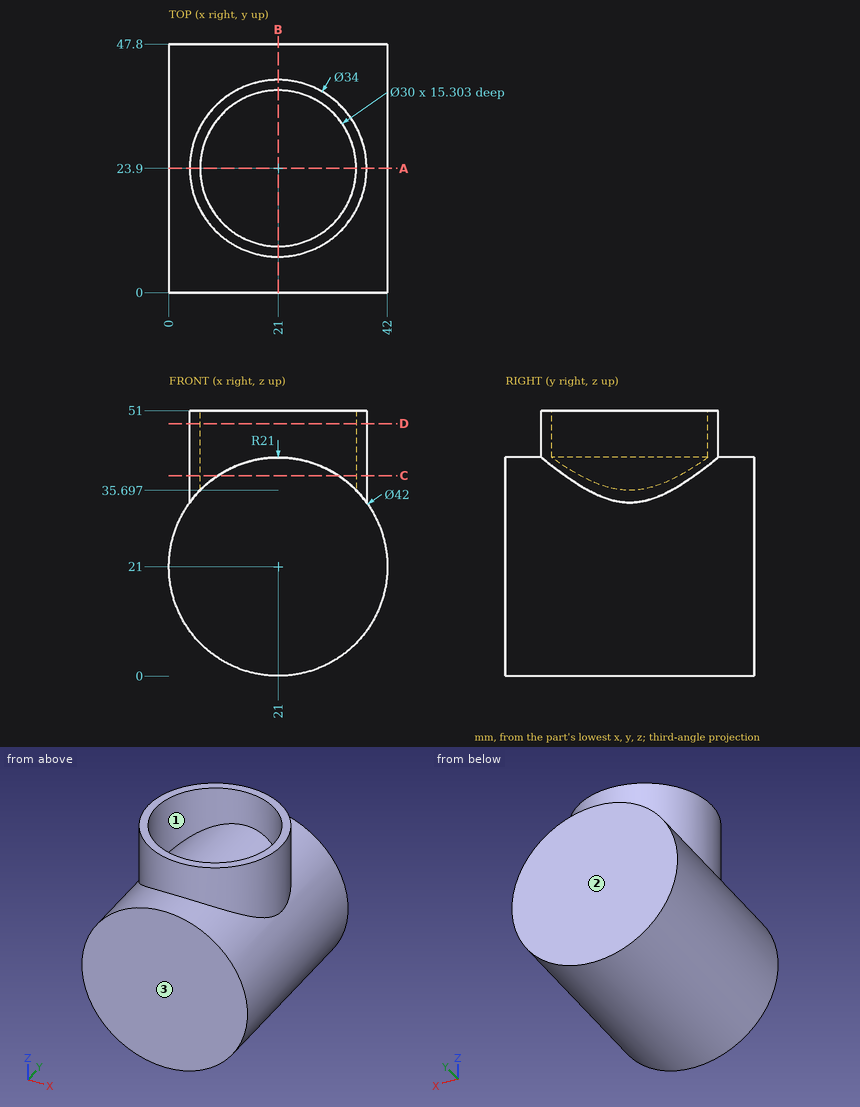
Design review of the part shown in the three views and the two pictorial views. Dimensions are in mm from the part's minimum x, y and z. Round coordinates to 2 decimals unless told otherwise and drop trailing zeros. Loops run counter-clockwise (first coordinate to the right, second up) from the corner with the lowest first, then second, coordinate; pieces in that order, holes last. Notation, with made-up numbers: (41.25, -19) -> (79.25, -19) arc R31 ccw to (79.25, 15) -> close; hole circle Ø8 at (-9, -14). An arc over 180 degrees is marked (long way). Use one line per item in the form item = value. Start each with the question number.
Q1. Wall thickness on line 1 along Y through (x, z) = (21, 43); line 2 along X through (y, z) = (18, 39); line 3 along Y through (x, z) = (32, 41): over which ranges is each line inside the solid? List them lowest first. Write a range as [from, to].
Q2. For pin 1 Ø2 at (x, y) = (6, 41.5) entering from +Z; pin 2 Ø1.5 at (y, z) = (35, 14.5) entering from +X; pin 3 Ø2 at (y, z) = (16, 34.5) entering from +X, all flat-tipped, find the tip position at first contact; note any pin that passes through.
Q3. We need section C-C on z = 38.5. Give the boundary of the cut face in (x, y), then the cut area to 3 significant figures.
Q4. We need section D-D on z = 48.5. Give the boundary of the cut face in (x, y), then the cut area to 3 significant figures.
Q5. Draft analysis for pull direction Y (two halves, no side actions). For the marked faces 1, 2 and 3, state which applies: +Y half, -Y half, draft (parallel to the pull), parting line (faces both ways), or undercut.
Q6. We need section A-A on y = 23.9. Give the boundary of the cut face in (x, z), then the cut area to 3 significant figures.
Q7. We need section B-B on x = 21. Give the boundary of the cut face in (y, z).
Calculated:
q1.line_1 = [6.9, 8.9], [38.9, 40.9]
q1.line_2 = [5.06, 7.21], [10.18, 31.82], [34.79, 36.94]
q1.line_3 = [10.94, 13.7], [34.1, 36.86]
q2.pin_1 = 36.65
q2.pin_2 = 41.2
q2.pin_3 = 37.87
q3.outline = (9.39, 0) -> (32.61, 0) -> (32.61, 11.48) arc R17 ccw to (32.61, 36.32) -> (32.61, 47.8) -> (9.39, 47.8) -> (9.39, 36.32) arc R17 ccw to (9.39, 11.48) -> close; hole (9.39, 14.4) -> (9.39, 33.4) arc R15 ccw to start; hole (32.61, 14.4) arc R15 ccw to (32.61, 33.4) -> close
q3.area = 1,210 mm²
q4.outline = circle Ø34 at (21, 23.9); hole circle Ø30 at (21, 23.9)
q4.area = 201 mm²
q5.face_1 = undercut
q5.face_2 = +Y half
q5.face_3 = -Y half
q6.outline = (4, 33.33) arc R21 ccw (long way) to (38, 33.33) -> (38, 51) -> (36, 51) -> (36, 35.7) arc R21 ccw to (6, 35.7) -> (6, 51) -> (4, 51) -> close
q6.area = 1,450 mm²
q7.outline = (0, 0) -> (47.8, 0) -> (47.8, 42) -> (40.9, 42) -> (40.9, 51) -> (38.9, 51) -> (38.9, 42) -> (8.9, 42) -> (8.9, 51) -> (6.9, 51) -> (6.9, 42) -> (0, 42) -> close
